Read the model definition and answer for the solid it produces. Units are mm, in the model's axes. A direction names the side the tool comes from. Coordinates: 2 decimals unless noted, no trailing zeros. Write each loop counter-clockwise with the first axis right and the second up, starting at its lowest first coordinate (ties: lowest second). Pieces come first, ordered by that corner, then holes.
(1) Given pin 1 (6 mm diameter, centred on x = -164, y = 274, fed in from +Z); pin 2 (7.5 mm diameter, centred on x = -41.57, y = 41.57, fed in from -Z); pin 3 (8 mm diameter, centred on x = -95, y = 305.5, fed in from +Z); pin 4 (10.5 mm diameter, centred on x = -161.63, y = 161.63, fed in from +Z), each flat-ended and moving along its own axis, determine where each tip first touches the part or whether it passes through.
(2) The part is cut by section A-A, the plane x = -106. Determine the outline of the cut face in (y, z), and give its area (3 significant figures).
(3) The part is cut by section C-C, the plane z = -187. Determine the outline of the cut face in (x, y).
(4) Straight lines are drawn through the part: line 1 along Z through (x, y) = (-126.5, 75); line 2 along Y through (x, z) = (-142, -82.5); line 3 along Y through (x, z) = (-120.5, -321). For each, find the intervals that lie inside material, in ascending order.
(5) The part is cut by section B-B, the plane y = 347.5. Determine the outline of the cut face in (x, z).
(6) Which of the six approach directions +Z, -Z, +X, -X, +Y, -Y give full straight-line access (tool end or side, diameter ignored) to faces 1 (the flat face through (-100, 0, -6)), 2 (the flat face through (-100, 100, -12.7))?
```python
from build123d import *

# Parameters (mm, degrees)
F0_W     = 203.2
F0_H     = 12.7
F1_DEPTH = 203.2
F3_D     = 6.5278


with BuildPart() as f1:
    # F0 (on Right) → F1 (new body)
    with BuildSketch(Plane.YZ):
        with Locations((101.6, -6.35)):
            Rectangle(F0_W, F0_H)
        Polygon((598.331269327, -395.131269327), (203.2, 0), (203.2, -12.7), (589.351013206, -404.1115254481), align=None)
    extrude(amount=-F1_DEPTH)

    # F3 (through all)
    with Locations(Plane.XY):
        with Locations((-161.6327916476, 161.6327916476), (-161.6327916476, 41.5672083524), (-41.5672083524, 41.5672083524), (-41.5672083524, 161.6327916476)):
            Hole(F3_D / 2)


solid = f1.part
```
Computed:
1. pin 1: stops at z = -67.8
1. pin 2: stops at z = -12.7
1. pin 3: stops at z = -98.3
1. pin 4: stops at z = 0
2. outline: (0, -12.7) - (203.2, -12.7) - (589.35, -404.11) - (598.33, -395.13) - (203.2, 0) - (0, 0) - close
2. area: 8,580 mm2
3. outline: (-203.2, 375.16) - (0, 375.16) - (0, 390.2) - (-203.2, 390.2) - close
4. line 1: z = -12.7 to 0
4. line 2: y = 272.06 to 285.7
4. line 3: y = 507.36 to 524.2
5. outline: (-203.2, -158.97) - (0, -158.97) - (0, -144.3) - (-203.2, -144.3) - close
6. face 1: +Z, -Z, +X, -X, -Y
6. face 2: -Z, +X, -X, -Y
